The listing builds one solid part. Answer for the finished solid, in the listing's coordinates (mm). A direction names the side the tool comes from. Coordinates: 2 decimals unless noted, no trailing zeros. Order: outer loops, then holes, each group sorted by start corner. A loop starts at its lowest first (then second) coordinate and runs counter-clockwise, first axis right, second up. Notation, with made-up numbers: (38.25, -7) -> (87.25, -7) arc R20 cw to (87.25, 31) -> close; hole circle Ø2 at (-9, 7.25). An arc over 180 degrees is marked (long way). Write item = value, one per line. Start each with the question number.
Autodesk Inventor part; units mm, degrees
ref_plane "YZ Plane" through (0, 0, 0) normal (1, 0, 0) x (0, 1, 0)
ref_plane "XZ Plane" through (0, 0, 0) normal (0, 1, 0) x (-1, 0, 0)
ref_plane "XY Plane" through (0, 0, 0) normal (0, 0, 1) x (1, 0, 0)
ref_plane "作業平面1" through (0, 0, 0) normal (0, 0, 1) x (1, 0, 0)
sketch "スケッチ1" plane through (0, 0, 0) normal (0, 0, 1) x (1, 0, 0)
  line L0 (-12.7, 11.83) -> (-12.7, 13.57)
  line L1 (12.3, -13.97) -> (10.56, -13.97)
  line L2 (12.7, -11.83) -> (12.7, -13.57)
  line L3 (-10, 10) -> (10, 10)
  line L4 (10, 10) -> (10, -10)
  line L5 (10, -10) -> (-10, -10)
  line L6 (-10, -10) -> (-10, 10)
  point P0 (0, 0)
  dimension "d35" = 10
  dimension "d36" = 20
  dimension "d37" = 10
  dimension "d39" = 20
extrude "押し出し1" add sketch "スケッチ1" against normal blind 1.6
sketch "スケッチ2" plane through (0, 0, 0) normal (0, 0, 1) x (1, 0, 0)
  circle A0 centre (-7, -5) radius 1.1
  circle A1 centre (7, 5) radius 1.1
  point P0 (0, 0)
  dimension "d2" = 2.2
  dimension "d3" = 2.2
  dimension "d4" = 7
  dimension "d7" = 7
  dimension "d43" = 5
  dimension "d44" = 5
extrude "押し出し2" cut sketch "スケッチ2" along normal mid plane 20
sketch "スケッチ5" plane through (0, 0, 0) normal (0, 0, 1) x (1, 0, 0)
  circle A0 centre (0, 0) radius 0.7
  line L0 (1.65, -8.8) -> (-1.65, -8.8)
  line L1 (-1.65, -8.8) -> (-1.65, -14.7)
  line L2 (-1.65, -14.7) -> (1.65, -14.7)
  line L3 (1.65, -14.7) -> (1.65, -8.8)
  dimension "d16" = 1.4
  dimension "d40" = 1.65
  dimension "d41" = 3.3
  dimension "d42" = 8.8
extrude "押し出し5" cut sketch "スケッチ5" against normal blind 20
properties part number "HbSensorBoard02" material "CFRP"
Item 1: Section D-D, the plane x = -1 is taken. Give the vertices of the cut face in (y, z).
Item 2: For a pull along X with two mould halves and no side action, classify faces 1 (the cylindrical face through (-0.7, 0, -0.8)), 2 (the flat face through (2, 0, -1.6)), 3 (the flat face through (-10, 0, -1)) as pulls with the +X half, pulls with the -X half, needs draft (parallel to the pull), parting line crosses it, or undercut.
Item 3: Section A-A, the plane y = 0 is taken. Give the vertices of the cut face in (x, z), then the cut area to 3 significant figures.
Item 4: Consider probe 1 along Y at (x, z) = (0, -0.85); probe 2 along Y at (x, z) = (-7, -0.9); probe 3 along Y at (x, z) = (0.75, -1.15). Determine where each line is inside the solid, lowest interval first.
Item 5: Section C-C, the plane z = -0.65 is taken. Give the vertices of the cut face in (x, y), then the cut area to 3 significant figures.
Item 6: Each of these flat-tipped pins is pushed along its axis until it touches: pin 1 (1.5 mm diameter, centred on x = 5.5, y = 5.5, fed in from +Z); pin 2 (0.8 mm diameter, centred on x = 0.5, z = -0.5, fed in from -Y). Where does it stop, or does it pass through?
Item 7: Which of the six approach directions +Z, -Z, +X, -X, +Y, -Y give full straight-line access (tool end or side, diameter ignored) to faces 4 (the flat face through (6, -10, -1)), 5 (the flat face through (1.65, -9, -1))?
Item 8: Section B-B, the plane x = 7 is taken. Give the vertices of the cut face in (y, z).
A:
q1.outline = (-8.8, -1.6) -> (10, -1.6) -> (10, 0) -> (-8.8, 0) -> close
q2.face_1 = undercut
q2.face_2 = needs draft
q2.face_3 = pulls with the -X half
q3.outline = (-10, -1.6) -> (-0.7, -1.6) -> (-0.7, 0) -> (-10, 0) -> close; (0.7, -1.6) -> (10, -1.6) -> (10, 0) -> (0.7, 0) -> close
q3.area = 29.8 mm^2
q4.probe_1 = -8.8 to -0.7, 0.7 to 10
q4.probe_2 = -10 to -6.1, -3.9 to 10
q4.probe_3 = -8.8 to 10
q5.outline = (-10, -10) -> (-1.65, -10) -> (-1.65, -8.8) -> (1.65, -8.8) -> (1.65, -10) -> (10, -10) -> (10, 10) -> (-10, 10) -> close; hole circle Ø2.2 at (-7, -5); hole circle Ø1.4 at (0, 0); hole circle Ø2.2 at (7, 5)
q5.area = 387 mm^2
q6.pin_1 = 0
q6.pin_2 = -8.8
q7.face_4 = +Z, -Z, +X, -X, -Y
q7.face_5 = +Z, -Z, -Y
q8.outline = (-10, -1.6) -> (3.9, -1.6) -> (3.9, 0) -> (-10, 0) -> close; (6.1, -1.6) -> (10, -1.6) -> (10, 0) -> (6.1, 0) -> close
